Geometry check sheet. Reference: the model listing, model coordinates, mm. Coordinates: 2 decimals unless noted, no trailing zeros. Order: outer loops, then holes, each group sorted by start corner. A loop starts at its lowest first (then second) coordinate and runs counter-clockwise, first axis right, second up. Notation, with made-up numbers: (36.5, 80.25) - (62.5, 80.25) arc R17 cw to (62.5, 110.25) - close; hole circle Ø9 at (-3, -10). An arc over 180 degrees is marked (long way). Put each result on its own line as item: value.
from build123d import *

# Parameters (mm, degrees)
SKETCH1_W           = 10
SKETCH1_H           = 10
BOSS_EXTRUDE1_DEPTH = 20
SKETCH3_R           = 1.25
CUT_EXTRUDE6_DEPTH  = 10


with BuildPart() as part:
    # Sketch1 → Boss-Extrude1 (new body)
    with BuildSketch(Plane.XY):
        Rectangle(SKETCH1_W, SKETCH1_H)
    extrude(amount=-BOSS_EXTRUDE1_DEPTH)

    # Sketch3 → Cut-Extrude6 (cut)
    with BuildSketch(Plane(origin=(5, 0, 0), x_dir=(0, 0, -1), z_dir=(1, 0, 0))):
        with Locations((7.5, 2)):
            Circle(SKETCH3_R)
    cut_extrude6 = extrude(amount=-CUT_EXTRUDE6_DEPTH, mode=Mode.SUBTRACT)

    # Mirror1: Cut-Extrude6 across plane
    add(cut_extrude6.mirror(Plane.ZX), mode=Mode.SUBTRACT)


solid = part.part
Q1. Section check D-D on y = 2.25. Record the boundary of the cut face in (x, z).
Answer block:
outline: (-5, -20) - (5, -20) - (5, -8.72) - (-5, -8.72) - close; (-5, -6.28) - (5, -6.28) - (5, 0) - (-5, 0) - close
Q2. Section check A-A on y = -2. Record the boundary of the cut face in (x, z).
Answer block:
outline: (-5, -20) - (5, -20) - (5, -8.75) - (-5, -8.75) - close; (-5, -6.25) - (5, -6.25) - (5, 0) - (-5, 0) - close
Q3. Section check B-B on z = -7.5. Record the boundary of the cut face in (x, y), then the cut area to 3 significant figures.
Answer block:
outline: (-5, -5) - (5, -5) - (5, -3.25) - (-5, -3.25) - close; (-5, -0.75) - (5, -0.75) - (5, 0.75) - (-5, 0.75) - close; (-5, 3.25) - (5, 3.25) - (5, 5) - (-5, 5) - close
area: 50.0 mm^2
Q4. Draft check along Z on faces 1 (the cylindrical face through (0.07, -2.05, -6.25)), 2 (the flat face through (0, 0, -20)), 3 (the flat face through (5, 0, -10)). Enter one of: pulls with the +Z half, pulls with the -Z half, needs draft (parallel to the pull), parting line crosses it, or undercut.
Answer block:
face 1: undercut
face 2: pulls with the -Z half
face 3: needs draft
Q5. Thickness scan on L1, parallel to Y at x = -1, z = -7.5; L2, parallel to Y at x = -2, z = -6.75; L3, parallel to Z at x = -1.25, y = -2. Record the ranges inside material, lowest first. Write a range as [from, to].
Answer block:
L1: y = [-5, -3.25], [-0.75, 0.75], [3.25, 5]
L2: y = [-5, -3], [-1, 1], [3, 5]
L3: z = [-20, -8.75], [-6.25, 0]
Q6. Section check C-C on x = 2.5. Record the boundary of the cut face in (y, z).
Answer block:
outline: (-5, -20) - (5, -20) - (5, 0) - (-5, 0) - close; hole circle Ø2.5 at (-2, -7.5); hole circle Ø2.5 at (2, -7.5)
